```python
from build123d import *

# Parameters (mm, degrees)
SKETCH1_W           = 12
SKETCH1_H           = 20
SKETCH1_R           = 1.6
BOSS_EXTRUDE1_DEPTH = 4
SKETCH18_W          = 5
SKETCH18_H          = 20
BOSS_EXTRUDE3_DEPTH = 100
CUT_EXTRUDE4_DEPTH  = 2
CUT_EXTRUDE5_DEPTH  = 5


with BuildPart() as part:
    # Sketch1 → Boss-Extrude1 (new body)
    with BuildSketch(Plane(origin=(0, 0, 0), x_dir=(1, 0, 0), z_dir=(0, 1, 0))):
        Rectangle(SKETCH1_W, SKETCH1_H)
        with Locations((-3, 7)):
            Circle(SKETCH1_R, mode=Mode.SUBTRACT)
        with Locations((-3, -7)):
            Circle(SKETCH1_R, mode=Mode.SUBTRACT)
    extrude(amount=BOSS_EXTRUDE1_DEPTH)

    # Sketch18 → Boss-Extrude3 (add)
    with BuildSketch(Plane(origin=(0, 4, 0), x_dir=(1, 0, 0), z_dir=(0, 1, 0))):
        with Locations((3.5, 0)):
            Rectangle(SKETCH18_W, SKETCH18_H)
    extrude(amount=BOSS_EXTRUDE3_DEPTH)

    # Sketch20 → Cut-Extrude4 (cut)
    with BuildSketch(Plane(origin=(0, 4, 0), x_dir=(1, 0, 0), z_dir=(0, 1, 0))):
        Polygon((-0.494371857, 5.523768453), (-0.468731907, 8.431821851), (-2.97436005, 9.908053397), (-5.505628143, 8.476231547), (-5.531268093, 5.568178149), (-3.02563995, 4.091946603), align=None)
        Polygon((-0.494371857, -8.441467238), (-0.498838682, -5.550795995), (-3.004466825, -4.109328757), (-5.505628143, -5.558532762), (-5.501161318, -8.449204005), (-2.995533175, -9.890671243), align=None)
    extrude(amount=-CUT_EXTRUDE4_DEPTH, mode=Mode.SUBTRACT)

    # Sketch21 → Cut-Extrude5 (cut)
    with BuildSketch(Plane(origin=(6, 0, 0), x_dir=(0, 0, -1), z_dir=(1, 0, 0))):
        with BuildLine():
            Line((-5.4, 100.304925489), (-5.4, 70.304925489))
            ThreePointArc((-5.4, 70.304925489), (-7, 68.704925489), (-8.6, 70.304925489))
            Line((-8.6, 70.304925489), (-8.6, 100.304925489))
            ThreePointArc((-8.6, 100.304925489), (-7, 101.904925489), (-5.4, 100.304925489))
        make_face()
        with BuildLine():
            Line((8.6, 100.170306459), (8.6, 70.170306459))
            ThreePointArc((8.6, 70.170306459), (7, 68.570306459), (5.4, 70.170306459))
            Line((5.4, 70.170306459), (5.4, 100.170306459))
            ThreePointArc((5.4, 100.170306459), (7, 101.770306459), (8.6, 100.170306459))
        make_face()
    extrude(amount=-CUT_EXTRUDE5_DEPTH, mode=Mode.SUBTRACT)


solid = part.part
```
Can you work these out from the model? Positions are in its coordinate system, mm. A direction names the side the tool comes from. Give positions to 0.01 mm unless a question says otherwise; leave off trailing zeros. Write each loop counter-clockwise with the first axis right and the second up, starting at its lowest first coordinate (ties: lowest second). Pieces come first, ordered by that corner, then holes. Notation, with made-up numbers: (57.25, 5.5) - (78.25, 5.5) arc R21 ccw to (78.25, 35.5) - close; hole circle Ø1 at (-4.5, 48). An arc over 180 degrees is marked (long way). Write item = value, one per line. Start each with the question number.
1. Imagine slicing it at B-B (z = 7). Please give me the cut outline in (x, y), and give its area (3 significant figures).
2. Imagine slicing it at D-D (z = 0.25). Please give me the cut outline in (x, y).
3. On a 3-axis mill with a long thin cutter (end or side, diameter ignored), from which of +Z, -Z, +X, -X, +Y, -Y can I reach the whole of each face in a straight line? I mean faces 4 (the face through (-6, 2, 0)), 5 (the face through (0, 0, 0)), 6 (the face through (-3, 4, 0)), 7 (the face through (-4.2, 3, 4.8)), 8 (the face through (3.54, 101.77, -6.96)). Say none if no direction works.
4. Imagine slicing it at C-C (y = 52.5). Please give me the cut outline in (x, z), and give its area (3 significant figures).
5. Please list where these lines run through material, in increasing order: line 1 (Z direction, x = 4.25, y = 91); line 2 (X direction, y = 0.7, z = 7); line 3 (Y direction, x = 3, z = 6.75).
6. Imagine slicing it at A-A (x = 3.5). Please give me the cut outline in (y, z).
7. Thinking about a two-plate mould opening in X: for faces 1 (the face through (4, 51, -10)), 2 (the face through (-3.35, 0.99, -5.44)), 3 (the face through (1, 53, 0)), which applies, released by +X, released by -X, zero draft, split by the parting line, or undercut?
8. For pin 1 (1 mm diameter, centred on y = 64, z = 2.5, fed in from -X); pin 2 (3 mm diameter, centred on x = -3, z = 7, fed in from -Y); pin 3 (5.5 mm diameter, centred on x = -3, z = 7, fed in from +Y); pin 4 (1.5 mm diameter, centred on x = -3, z = -6, fed in from +Y), each with a flat end and sliding along its axis, tell me the tip position at first contact or that it passes through.
Worked answers:
q1.outline = (-6, 0) - (-4.6, 0) - (-4.6, 2) - (-5.5, 2) - (-5.5, 4) - (-6, 4) - close; (-1.4, 0) - (6, 0) - (6, 68.7) - (1, 68.7) - (1, 4) - (-0.5, 4) - (-0.5, 2) - (-1.4, 2) - close; (1, 101.9) - (6, 101.9) - (6, 104) - (1, 104) - close
q1.area = 366 mm2
q2.outline = (-6, 0) - (6, 0) - (6, 104) - (1, 104) - (1, 4) - (-6, 4) - close
q3.face_4 = +Z, -Z, -X, +Y, -Y
q3.face_5 = +Z, -Z, +X, -X, -Y
q3.face_6 = +Z, -Z, -X, +Y
q3.face_7 = +Y
q3.face_8 = +X, -X
q4.outline = (1, -10) - (6, -10) - (6, 10) - (1, 10) - close
q4.area = 100 mm2
q5.line_1 = -10 to -8.6, -5.4 to 5.4, 8.6 to 10
q5.line_2 = -6 to -4.6, -1.4 to 6
q5.line_3 = 0 to 68.72, 101.89 to 104
q6.outline = (0, -10) - (104, -10) - (104, 10) - (0, 10) - close; hole (70.17, -8.6) - (100.17, -8.6) arc R1.6 ccw to (100.17, -5.4) - (70.17, -5.4) arc R1.6 ccw to start; hole (70.3, 5.4) - (100.3, 5.4) arc R1.6 ccw to (100.3, 8.6) - (70.3, 8.6) arc R1.6 ccw to start
q7.face_1 = zero draft
q7.face_2 = undercut
q7.face_3 = released by -X
q8.pin_1 = 1
q8.pin_2 = through
q8.pin_3 = 4
q8.pin_4 = 2
